```python
from build123d import *

# Parameters (mm, degrees)
SKETCH1_W               = 8
SKETCH1_H               = 3.5
BOSS_EXTRUDE1_DEPTH     = 5
SKETCH2_W               = 8
SKETCH2_H               = 3.5
BOSS_EXTRUDE2_DEPTH     = 8
CHAMFER1_SIZE           = 0.5
CUT_EXTRUDE1_DEPTH      = 15.044571905
CUT_EXTRUDE1_DEPTH_BACK = 15.044571905
SKETCH3_R               = 1.2


with BuildPart() as part:
    # Sketch1 → Boss-Extrude1 (new, symmetric)
    with BuildSketch(Plane.XY):
        Rectangle(SKETCH1_W, SKETCH1_H)
    extrude(amount=BOSS_EXTRUDE1_DEPTH, both=True)

    # Sketch2 → Boss-Extrude2 (add)
    with BuildSketch(Plane(origin=(0, 0, -5), x_dir=(-1, 0, 0), z_dir=(0, 0, -1))):
        Rectangle(SKETCH2_W, SKETCH2_H)
    boss_extrude2 = extrude(amount=BOSS_EXTRUDE2_DEPTH)

    # Mirror1: Boss-Extrude2 across plane
    add(boss_extrude2.mirror(Plane.XY))

    # Chamfer1
    chamfer1_edges = [part.edges().sort_by_distance(p)[0] for p in [
        (0, 1.75, -13),
        (0, -1.75, -13),
        (0, -1.75, 13),
        (0, 1.75, 13),
        (4, -1.75, 0),
        (-4, -1.75, 0),
        (-4, 1.75, 0),
        (4, 1.75, 0),
    ]]
    chamfer(chamfer1_edges, length=CHAMFER1_SIZE)

    # Sketch3 → Cut-Extrude1 (cut, two sides: drawn at the far end of the back side and taken through both)
    with BuildSketch(Plane(origin=(0, 1.75, 0), x_dir=(1, 0, 0), z_dir=(0, 1, 0)).offset(-CUT_EXTRUDE1_DEPTH_BACK)):
        with Locations(Location((0, -9, 0), (0, 0, 270))):
            Circle(SKETCH3_R)
        with Locations(Location((0, 9, 0), (0, 0, 270))):
            Circle(SKETCH3_R)
    extrude(amount=CUT_EXTRUDE1_DEPTH + CUT_EXTRUDE1_DEPTH_BACK, mode=Mode.SUBTRACT)


solid = part.part
```
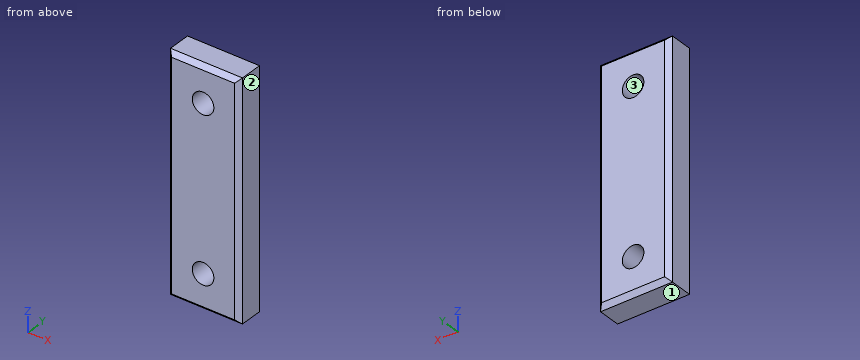
Here's how the part is built. I have some questions about the finished solid (model axes, mm). Face numbers are marked on the shaded views. Give positions to 0.01 mm unless a question says otherwise; leave off trailing zeros. Write each loop counter-clockwise with the first axis right and the second up, starting at its lowest first coordinate (ties: lowest second). Pieces come first, ordered by that corner, then holes.
(1) Imagine slicing it at D-D, the plane z = -6. Write out the boundary of the cut face in (x, y), and give its area (3 significant figures).
Output values:
outline: (-4, -1.25) - (-3.5, -1.75) - (3.5, -1.75) - (4, -1.25) - (4, 1.25) - (3.5, 1.75) - (-3.5, 1.75) - (-4, 1.25) - close
area: 27.5 mm2
(2) If I drill on L1, parallel to Z at x = 0, y = -0.15; L2, parallel to X at y = 0.25, z = -9; L3, parallel to Z at x = 0.5, y = 0.05, over which ranges is the centre line in solid material (lowest first)?
Output values:
L1: z = -13 to -10.2, -7.8 to 7.8, 10.2 to 13
L2: x = -4 to -1.2, 1.2 to 4
L3: z = -13 to -10.09, -7.91 to 7.91, 10.09 to 13
(3) Imagine slicing it at B-B, the plane z = 9. Write out the boundary of the cut face in (x, y), and give its area (3 significant figures).
Output values:
outline: (-4, -1.25) - (-3.5, -1.75) - (-1.2, -1.75) - (-1.2, 1.75) - (-3.5, 1.75) - (-4, 1.25) - close; (1.2, -1.75) - (3.5, -1.75) - (4, -1.25) - (4, 1.25) - (3.5, 1.75) - (1.2, 1.75) - close
area: 19.1 mm2
(4) Thinking about a two-plate mould opening in X: for the marked faces 1, 2 and 3, which applies, pulls with the +X half, pulls with the -X half, needs draft (parallel to the pull), parting line crosses it, or undercut?
Output values:
face 1: needs draft
face 2: pulls with the +X half
face 3: undercut
(5) Imagine slicing it at A-A, the plane x = 0. Write out the boundary of the cut face in (y, z).
Output values:
outline: (-1.75, -12.5) - (-1.25, -13) - (1.25, -13) - (1.75, -12.5) - (1.75, -10.2) - (-1.75, -10.2) - close; (-1.75, -7.8) - (1.75, -7.8) - (1.75, 7.8) - (-1.75, 7.8) - close; (-1.75, 10.2) - (1.75, 10.2) - (1.75, 12.5) - (1.25, 13) - (-1.25, 13) - (-1.75, 12.5) - close
(6) Imagine slicing it at C-C, the plane y = -1.5. Write out the boundary of the cut face in (x, z), and give its area (3 significant figures).
Output values:
outline: (-3.75, -12.75) - (3.75, -12.75) - (3.75, 12.75) - (-3.75, 12.75) - close; hole circle Ø2.4 at (0, -9); hole circle Ø2.4 at (0, 9)
area: 182 mm2
